Could you check a few things on this model? Use its own coordinates, in mm. A direction names the side the tool comes from. Round coordinates to 2 decimals unless told otherwise and drop trailing zeros. Order: outer loops, then holes, each group sorted by start corner. A loop starts at its lowest first (then second) coordinate and runs counter-clockwise, first axis right, second up. Notation, with made-up numbers: M 86,-36 L 132,-36 A19 cw 132,-31 Z; hole C 71,46.5 d6. An arc over 180 degrees is marked long. Write each question's results on one line, items separated by ' | '. Start each with the question number.
1. For faces 1 (the flat face through (5, -209.55, 5)), 2 (the flat face through (249, -234.95, 5)), 3 (the flat face through (89, -10.16, 5)), which set-ups out of +Z, -Z, +X, -X, +Y, -Y let a thin tool reach every point of the face, with its end or its side?
2. Suppose I cut it at B-B on y = -154. Write out the boundary of the cut face in (x, z), and give its area (3 significant figures).
3. Please list where these lines run through material, in increasing order: L1, parallel to Y at x = 62, z = 8; L2, parallel to X at y = -155, z = 2.75.
4. I'm going to push a flat-ended pin straight in: pin 1 (3 mm diameter, centred on y = -27.5, z = 5.5, fed in from +X). Where does the tip first touch, or does it pass through?
5. We'd pull the mould along X, two halves only. Please class faces 4 (the flat face through (243.84, -178, 5)), 5 (the flat face through (5, -57.15, 5)), 6 (the flat face through (191, -10.16, 5)), 7 (the flat face through (31.75, -249, 5)): released by +X, released by -X, zero draft, split by the parting line, or undercut.
6. Suppose I cut it at A-A on x = 65.5. Write out the boundary of the cut face in (y, z).
from build123d import *

# Parameters (mm, degrees)
F1_DEPTH = 10.16


with BuildPart() as f1:
    # F0 (on Top) → F1 (new body)
    with BuildSketch(Plane.XY):
        Polygon((31.75, 0), (0, 0), (0, -19.05), (10.16, -19.05), (10.16, -31.75), (0, -31.75), (0, -44.45), (10.16, -44.45), (10.16, -57.15), (0, -57.15), (0, -69.85), (10.16, -69.85), (10.16, -82.55), (0, -82.55), (0, -95.25), (10.16, -95.25), (10.16, -107.95), (0, -107.95), (0, -120.65), (10.16, -120.65), (10.16, -133.35), (0, -133.35), (0, -146.05), (10.16, -146.05), (10.16, -158.75), (0, -158.75), (0, -171.45), (10.16, -171.45), (10.16, -184.15), (0, -184.15), (0, -196.85), (10.16, -196.85), (10.16, -209.55), (0, -209.55), (0, -222.25), (10.16, -222.25), (10.16, -234.95), (0, -234.95), (0, -254), (31.75, -254), (31.75, -243.84), (44.45, -243.84), (44.45, -254), (57.15, -254), (57.15, -243.84), (69.85, -243.84), (69.85, -254), (82.55, -254), (82.55, -243.84), (95.25, -243.84), (95.25, -254), (107.95, -254), (107.95, -243.84), (120.65, -243.84), (120.65, -254), (133.35, -254), (133.35, -243.84), (146.05, -243.84), (146.05, -254), (158.75, -254), (158.75, -243.84), (171.45, -243.84), (171.45, -254), (184.15, -254), (184.15, -243.84), (196.85, -243.84), (196.85, -254), (209.55, -254), (209.55, -243.84), (222.25, -243.84), (222.25, -254), (254, -254), (254, -234.95), (243.84, -234.95), (243.84, -222.25), (254, -222.25), (254, -209.55), (243.84, -209.55), (243.84, -196.85), (254, -196.85), (254, -184.15), (243.84, -184.15), (243.84, -171.45), (254, -171.45), (254, -158.75), (243.84, -158.75), (243.84, -146.05), (254, -146.05), (254, -133.35), (243.84, -133.35), (243.84, -120.65), (254, -120.65), (254, -107.95), (243.84, -107.95), (243.84, -95.25), (254, -95.25), (254, -82.55), (243.84, -82.55), (243.84, -69.85), (254, -69.85), (254, -57.15), (243.84, -57.15), (243.84, -44.45), (254, -44.45), (254, -31.75), (243.84, -31.75), (243.84, -19.05), (254, -19.05), (254, 0), (222.25, 0), (222.25, -10.16), (209.55, -10.16), (209.55, 0), (196.85, 0), (196.85, -10.16), (184.15, -10.16), (184.15, 0), (171.45, 0), (171.45, -10.16), (158.75, -10.16), (158.75, 0), (146.05, 0), (146.05, -10.16), (133.35, -10.16), (133.35, 0), (120.65, 0), (120.65, -10.16), (107.95, -10.16), (107.95, 0), (95.25, 0), (95.25, -10.16), (82.55, -10.16), (82.55, 0), (69.85, 0), (69.85, -10.16), (57.15, -10.16), (57.15, 0), (44.45, 0), (44.45, -10.16), (31.75, -10.16), align=None)
    extrude(amount=F1_DEPTH)


solid = f1.part
Filled sheet:
1) face 1: +Z, -Z, -X | face 2: +Z, -Z, +X | face 3: +Z, -Z, +Y
2) outline: M 10.16,0 L 243.84,0 L 243.84,10.16 L 10.16,10.16 Z | area: 2,370 mm^2
3) L1: y = -243.84 to -10.16 | L2: x = 10.16 to 243.84
4) pin 1: stops at x = 243.84
5) face 4: released by +X | face 5: zero draft | face 6: undercut | face 7: undercut
6) outline: M -243.84,0 L -10.16,0 L -10.16,10.16 L -243.84,10.16 Z
